Read the model definition and answer for the solid it produces. Units are mm, in the model's axes. Coordinates: 2 decimals unless noted, no trailing zeros. Loops run counter-clockwise (first coordinate to the right, second up) from the corner with the lowest first, then second, coordinate; pieces in that order, holes last. Notation, with made-up numbers: (-38, 66) - (7, 66) arc R13 ccw to (7, 89) - close; hole circle Ø2 at (80.25, 17.25). An arc over 180 degrees is marked (long way). Use one line per item in the form item = value. Start each with the question number.
1) A cutting plane is placed at B-B (x = 1.1). Give the vertices of the cut face in (y, z), and give its area (3 significant figures).
2) A cutting plane is placed at A-A (y = 0). Give the vertices of the cut face in (x, z).
3) A cutting plane is placed at D-D (x = 1.95). Give the vertices of the cut face in (y, z), and give its area (3 significant figures).
4) A cutting plane is placed at C-C (z = 2). Give the vertices of the cut face in (x, y), and give its area (3 significant figures).
5) Consider line 1 (Y direction, x = 0, z = 3); line 2 (X direction, y = 0.85, z = 1.25); line 3 (X direction, y = 0.55, z = 5). Determine where each line is inside the solid, lowest interval first.
6) The mould has two halves that part along Y. Classify faces 1 (the face through (-1, -1, 0)), 2 (the face through (-1.976, -1.515, 5.181)), 3 (the face through (0, 0, 7)): released by +Y, released by -Y, zero draft, split by the parting line, or undercut.
7) Each of these flat-tipped pins is pushed along its axis until it touches: P1, Ø0.8, axis at x = 0.5, y = 0, coming from the -Z side; P2, Ø1.5, axis at x = 1.5, z = 10, coming from the -Y side; P3, Ø1.5, axis at x = -2, y = -1.5, coming from the +Z side. Where does it stop, or does it pass through?
from build123d import *

# Parameters (mm, degrees)
F0_R     = 2.49
F1_DEPTH = 13
F2_R     = 1.25
F3_DEPTH = 7
F4_R     = 2.49


with BuildPart() as f1:
    # F0 (on Top) → F1 (new body)
    with BuildSketch(Plane.XY):
        Circle(F0_R)
    extrude(amount=F1_DEPTH)

    # F2 (on face) → F3 (cut)
    with BuildSketch(Plane(origin=(0, 0, 0), x_dir=(1, 0, 0), z_dir=(0, 0, -1))):
        Circle(F2_R)
    extrude(amount=-F3_DEPTH, mode=Mode.SUBTRACT)

    # F4
    f4_edges = [f1.edges().sort_by_distance(p)[0] for p in [
        (-2.49, 0, 13),
    ]]
    fillet(f4_edges, radius=F4_R)


solid = f1.part
Found:
q1.outline = (-2.23, 0) - (-0.59, 0) - (-0.59, 7) - (0.59, 7) - (0.59, 0) - (2.23, 0) - (2.23, 10.51) arc R2.23 ccw to (-2.23, 10.51) - close
q1.area = 46.5 mm^2
q2.outline = (-2.49, 0) - (-1.25, 0) - (-1.25, 7) - (1.25, 7) - (1.25, 0) - (2.49, 0) - (2.49, 10.51) arc R2.49 ccw to (-2.49, 10.51) - close
q3.outline = (-1.55, 0) - (1.55, 0) - (1.55, 10.51) arc R1.55 ccw to (-1.55, 10.51) - close
q3.area = 36.3 mm^2
q4.outline = circle Ø4.98 at (0, 0); hole circle Ø2.5 at (0, 0)
q4.area = 14.6 mm^2
q5.line_1 = -2.49 to -1.25, 1.25 to 2.49
q5.line_2 = -2.34 to -0.92, 0.92 to 2.34
q5.line_3 = -2.43 to -1.12, 1.12 to 2.43
q6.face_1 = zero draft
q6.face_2 = split by the parting line
q6.face_3 = undercut
q7.P1 = 7
q7.P2 = -2.37
q7.P3 = 12.28
